Here's the drawing with two shaded views (mm, measured from the low corner). I have some questions. A direction names the side the tool comes from. Round coordinates to 2 decimals unless told otherwise and drop trailing zeros. Order: outer loops, then holes, each group sorted by start corner. A loop starts at its lowest first (then second) coordinate and runs counter-clockwise, first axis right, second up.
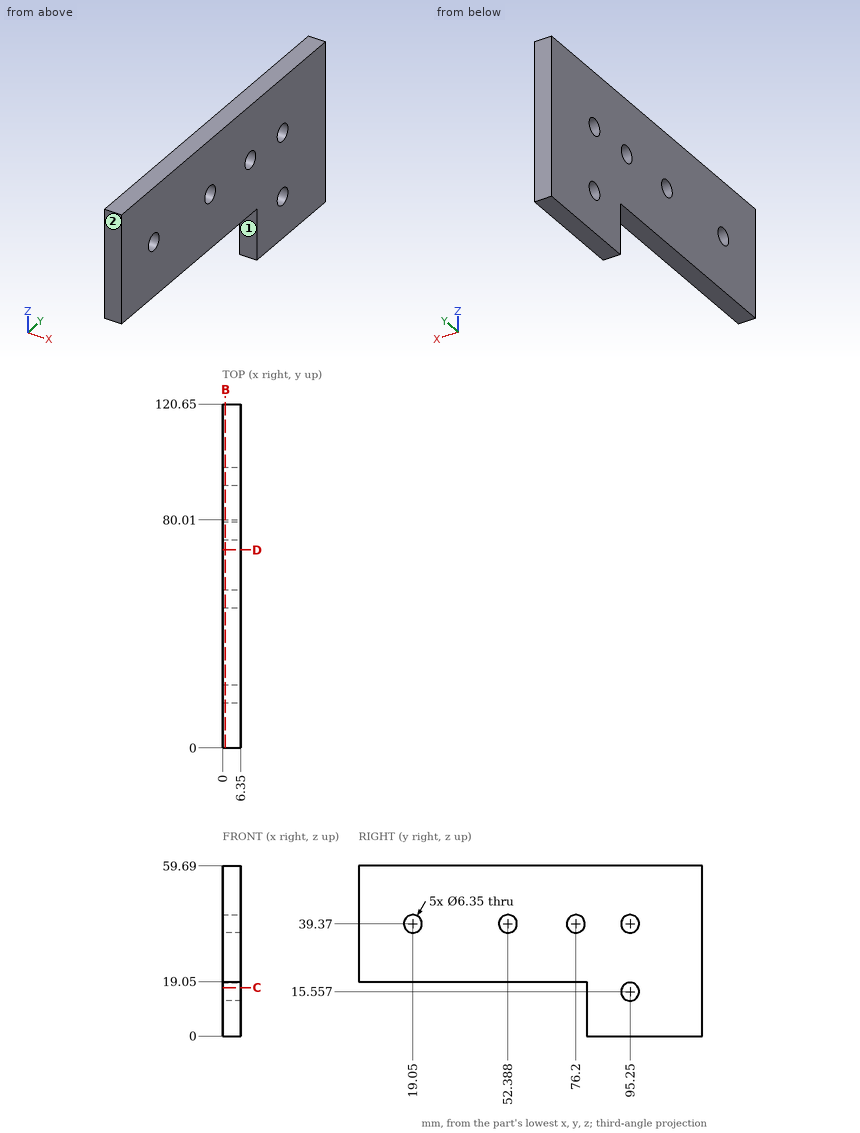
1. If we section it at B-B, the plane x = 1: State how many separate pieces and enclosed holes the cut face has, and give its area (3 significant figures).
Evaluation:
separate pieces: 1
enclosed holes: 5
area: 5,520 mm2
2. If we section it at D-D, the plane y = 69.5: Write out the boundary of the cut face in (x, z), and give its area (3 significant figures).
Evaluation:
outline: (0, 19.05) - (6.35, 19.05) - (6.35, 59.69) - (0, 59.69) - close
area: 258 mm2
3. If we section it at C-C, the plane z = 17: Write out the boundary of the cut face in (x, y).
Evaluation:
outline: (0, 80.01) - (6.35, 80.01) - (6.35, 92.42) - (0, 92.42) - close; (0, 98.08) - (6.35, 98.08) - (6.35, 120.65) - (0, 120.65) - close
4. I'm going to push flat-ended pins straight in: P1, Ø4, axis at y = 76.2, z = 39.37, coming from the -X side; P2, Ø1.9, axis at x = 2, z = 12.5, coming from the -Y side. Where does each tip first touch, or does it pass through?
Evaluation:
P1: passes through
P2: stops at y = 80.01
5. On a 3-axis mill with a long thin cutter (end or side, diameter ignored), from which of +Z, -Z, +X, -X, +Y, -Y can I reach the whole of each face in a straight line? I mean the marked faces 1 and 2. Say none if no direction works.
Evaluation:
face 1: -Z, +X, -X, -Y
face 2: +Z, -Z, +X, -X, -Y
6. I need wall thicknesses on probe 1 along Z at (x, y) = (2.75, 95.5) (1 decimal); probe 2 along Z at (x, y) = (3.25, 62); probe 3 along Z at (x, y) = (5.75, 52). Which ranges of each line are inside material? Lowest first, please.
Evaluation:
probe 1: z = 0 to 12.4, 18.7 to 36.2, 42.5 to 59.7
probe 2: z = 19.05 to 59.69
probe 3: z = 19.05 to 36.22, 42.52 to 59.69
